```python
from build123d import *

# Parameters (mm, degrees)
CROQUIS1_W              = 130
CROQUIS1_H              = 110
CROQUIS1_W_2            = 80
CROQUIS1_H_2            = 60
SALIENTE_EXTRUIR1_DEPTH = 2
CROQUIS2_R              = 1.5
CORTAR_EXTRUIR2_DEPTH   = 171.305607659


with BuildPart() as part:
    # Croquis1 → Saliente-Extruir1 (new body)
    with BuildSketch(Plane.XY):
        with Locations((65, 55)):
            Rectangle(CROQUIS1_W, CROQUIS1_H)
        with Locations((65, 55)):
            Rectangle(CROQUIS1_W_2, CROQUIS1_H_2, mode=Mode.SUBTRACT)
    extrude(amount=SALIENTE_EXTRUIR1_DEPTH)

    # Croquis2 → Cortar-Extruir2 (cut, through all)
    with BuildSketch(Plane.XY):
        with Locations((12.5, 97.5)):
            Circle(CROQUIS2_R)
        with Locations((47.5, 97.5)):
            Circle(CROQUIS2_R)
        with Locations((82.5, 97.5)):
            Circle(CROQUIS2_R)
        with Locations((117.5, 97.5)):
            Circle(CROQUIS2_R)
        with Locations((12.5, 69.17)):
            Circle(CROQUIS2_R)
        with Locations((12.5, 40.84)):
            Circle(CROQUIS2_R)
        with Locations(Location((117.5, 12.5, 0), (0, 0, 180))):
            Circle(CROQUIS2_R)
        with Locations(Location((82.5, 12.5, 0), (0, 0, 180))):
            Circle(CROQUIS2_R)
        with Locations(Location((47.5, 12.5, 0), (0, 0, 180))):
            Circle(CROQUIS2_R)
        with Locations(Location((12.5, 12.5, 0), (0, 0, 180))):
            Circle(CROQUIS2_R)
        with Locations(Location((117.5, 40.84, 0), (0, 0, 180))):
            Circle(CROQUIS2_R)
        with Locations(Location((117.5, 69.17, 0), (0, 0, 180))):
            Circle(CROQUIS2_R)
    extrude(amount=CORTAR_EXTRUIR2_DEPTH, mode=Mode.SUBTRACT)


solid = part.part
```
Could you check a few things on this model? Use its own coordinates, in mm. Round coordinates to 2 decimals unless told otherwise and drop trailing zeros. Loops run counter-clockwise (first coordinate to the right, second up) from the corner with the lowest first, then second, coordinate; pieces in that order, holes last. Notation, with made-up numbers: M 13.25,49 L 71.25,49 A10 ccw 71.25,65 Z; hole C 82,46 d11. An arc over 180 degrees is marked long. Answer as CSV lines item,"result".
1) Imagine slicing it at B-B on z = 1.7. Count the separate pieces of the cut face and the enclosed holes in it, and give its area (3 significant figures).
From the geometry:
separate pieces,"1"
enclosed holes,"13"
area,"9,420 mm^2"
2) Imagine slicing it at A-A on x = 47.5. List the corners of the cut face in (y, z) for me, and give its area (3 significant figures).
From the geometry:
outline,"M 0,0 L 11,0 L 11,2 L 0,2 Z; M 14,0 L 25,0 L 25,2 L 14,2 Z; M 85,0 L 96,0 L 96,2 L 85,2 Z; M 99,0 L 110,0 L 110,2 L 99,2 Z"
area,"88.0 mm^2"
3) We'd pull the mould along Y, two halves only. Please class faces 1 (the flat face through (64, 92, 0)), 2 (the cylindrical face through (119, 40.8, 1)): released by +Y, released by -Y, zero draft, split by the parting line, or undercut.
From the geometry:
face 1,"zero draft"
face 2,"undercut"
4) Imagine slicing it at D-D on x = 117.5. List the corners of the cut face in (y, z) for me.
From the geometry:
outline,"M 0,0 L 11,0 L 11,2 L 0,2 Z; M 14,0 L 39.34,0 L 39.34,2 L 14,2 Z; M 42.34,0 L 67.67,0 L 67.67,2 L 42.34,2 Z; M 70.67,0 L 96,0 L 96,2 L 70.67,2 Z; M 99,0 L 110,0 L 110,2 L 99,2 Z"
5) Imagine slicing it at C-C on y = 40.84. List the corners of the cut face in (x, z) for me, and give its area (3 significant figures).
From the geometry:
outline,"M 0,0 L 11,0 L 11,2 L 0,2 Z; M 14,0 L 25,0 L 25,2 L 14,2 Z; M 105,0 L 116,0 L 116,2 L 105,2 Z; M 119,0 L 130,0 L 130,2 L 119,2 Z"
area,"88.0 mm^2"
6) If I drill on probe 1 along X at (y, z) = (12.5, 1.2); probe 2 along Y at (x, z) = (47.5, 1.55); probe 3 along Y at (x, z) = (117.5, 1), over which ranges is the centre line in solid material (lowest first)?
From the geometry:
probe 1,"0 to 11, 14 to 46, 49 to 81, 84 to 116, 119 to 130"
probe 2,"0 to 11, 14 to 25, 85 to 96, 99 to 110"
probe 3,"0 to 11, 14 to 39.34, 42.34 to 67.67, 70.67 to 96, 99 to 110"
